from build123d import *

# Parameters (mm, degrees)
EXTRUDE_1_DEPTH      = 10.8
SKETCH_2_R           = 1
EXTRUDE_2_DEPTH      = 0.8
SKETCH_3_W           = 1.7
SKETCH_3_H           = 8.1
CUT_EXTRUDE_1_DEPTH  = 17.8
EXTRUDE_START        = -4.5
EXTRUDE_3_DEPTH      = 4.5
SKETCH_5_W           = 8.4
SKETCH_5_H           = 0.05
CUT_EXTRUDE_2_DEPTH  = 1
SKETCH_6_R           = 1
CUT_EXTRUDE_3_DEPTH  = 8
CUT_EXTRUDE_4_DEPTH  = 1.2
SKETCH_8_W           = 2.8
SKETCH_8_H           = 0.608363533
EXTRUDE_4_DEPTH      = 0.1
EXTRUDE_START_2      = 2.5
EXTRUDE_5_DEPTH      = 2.5
SKETCH_10_W          = 8.4
SKETCH_10_H          = 1.7
CUT_EXTRUDE_5_DEPTH  = 0.05
FILLET_1_R           = 1.4
SKETCH_11_W          = 0.05
SKETCH_11_H          = 5.83834946
SKETCH_11_H_2        = 5.828769054
CUT_EXTRUDE_8_DEPTH  = 0.05
CUT_EXTRUDE_9_DEPTH  = 4
SKETCH_13_W          = 0.5
SKETCH_13_H          = 5.54
EXTRUDE_6_DEPTH      = 1.45
FILLET_2_R           = 1
CUT_EXTRUDE_START    = -8.12
CUT_EXTRUDE_10_DEPTH = 8.12
SKETCH_15_W          = 3
SKETCH_15_H          = 0.25
CUT_EXTRUDE_11_DEPTH = 8.12
SKETCH_16_W          = 0.5
SKETCH_16_H          = 0.25
EXTRUDE_7_DEPTH      = 3
FILLET_3_R           = 0.5
FILLET_4_R           = 0.75


with BuildPart() as part:
    # Эскиз1 → Бобышка-Вытянуть1 (new body)
    with BuildSketch(Plane.XY):
        Polygon((7.4, 0), (8.4, 1), (8.4, 12.6), (0, 12.6), (0, 1), (1, 0), align=None)
    extrude(amount=EXTRUDE_1_DEPTH)

    # Эскиз2 → Бобышка-Вытянуть2 (add)
    with BuildSketch(Plane(origin=(0, 0, 0), x_dir=(-1, 0, 0), z_dir=(0, 0, -1))):
        with Locations((-4.2, 10.3)):
            Circle(SKETCH_2_R)
        with Locations((-4.2, 3.9)):
            Circle(SKETCH_2_R)
    extrude(amount=EXTRUDE_2_DEPTH)

    # Эскиз3 → Вырез-Вытянуть1 (cut)
    with BuildSketch(Plane(origin=(8.4, 0, 0), x_dir=(0, 0, -1), z_dir=(1, 0, 0))):
        with Locations((-4.75, 4.05)):
            Rectangle(SKETCH_3_W, SKETCH_3_H)
    extrude(amount=-CUT_EXTRUDE_1_DEPTH, mode=Mode.SUBTRACT)

    # Эскиз4 → Бобышка-Вытянуть3 (add)
    with BuildSketch(Plane(origin=(0, 12.6, 0), x_dir=(1, 0, 0), z_dir=(0, 1, 0)).offset(EXTRUDE_START)):
        with BuildLine():
            Line((9.1, -10.8), (-0.7, -10.8))
            Line((-0.7, -10.8), (-0.7, -2.8))
            ThreePointArc((-0.7, -2.8), (-0.992893219, -2.092893219), (-1.7, -1.8))
            Line((-1.7, -1.8), (-5.9, -1.8))
            Line((-5.9, -1.8), (-5.9, 0))
            Line((-5.9, 0), (14.3, 0))
            Line((14.3, 0), (14.3, -1.8))
            Line((14.3, -1.8), (10.1, -1.8))
            ThreePointArc((10.1, -1.8), (9.392893219, -2.092893219), (9.1, -2.8))
            Line((9.1, -2.8), (9.1, -10.8))
        make_face()
    extrude(amount=EXTRUDE_3_DEPTH)

    # Эскиз5 → Вырез-Вытянуть2 (cut)
    with BuildSketch(Plane.XY.offset(10.8)):
        with Locations((4.2, 8.075)):
            Rectangle(SKETCH_5_W, SKETCH_5_H)
    extrude(amount=-CUT_EXTRUDE_2_DEPTH, mode=Mode.SUBTRACT)

    # Эскиз6 → Вырез-Вытянуть3 (cut)
    with BuildSketch(Plane.XY.offset(10.8)):
        with Locations((4.2, 4)):
            Circle(SKETCH_6_R)
    extrude(amount=-CUT_EXTRUDE_3_DEPTH, mode=Mode.SUBTRACT)

    # Эскиз7 → Вырез-Вытянуть4 (cut)
    with BuildSketch(Plane(origin=(0, 12.6, 0), x_dir=(1, 0, 0), z_dir=(0, 1, 0))):
        with BuildLine():
            Line((8.6, 0), (8.6, -7.112411136))
            ThreePointArc((8.6, -7.112411136), (8.468198052, -7.430609188), (8.15, -7.562411136))
            Line((8.15, -7.562411136), (7.983405928, -7.562411136))
            ThreePointArc((7.983405928, -7.562411136), (7.691564003, -7.454943311), (7.539115931, -7.183870205))
            Line((7.539115931, -7.183870205), (7.049736844, -4.141202068))
            ThreePointArc((7.049736844, -4.141202068), (6.710963351, -3.53881739), (6.062425739, -3.3))
            Line((6.062425739, -3.3), (2.361664993, -3.3))
            ThreePointArc((2.361664993, -3.3), (1.71573807, -3.536600753), (1.37546474, -4.13444318))
            Line((1.37546474, -4.13444318), (0.863036378, -7.186911705))
            ThreePointArc((0.863036378, -7.186911705), (0.709913379, -7.455940797), (0.419246264, -7.562411136))
            Line((0.419246264, -7.562411136), (0.25, -7.562411136))
            ThreePointArc((0.25, -7.562411136), (-0.068198052, -7.430609188), (-0.2, -7.112411136))
            Line((-0.2, -7.112411136), (-0.2, 0))
            Line((-0.2, 0), (8.6, 0))
        make_face()
        with BuildLine():
            Line((4.2, -10.8), (5.6, -10.8))
            Line((5.6, -10.8), (5.6, -5.056380156))
            ThreePointArc((5.6, -5.056380156), (5.453553391, -4.702826765), (5.1, -4.556380156))
            Line((5.1, -4.556380156), (3.3, -4.556380156))
            ThreePointArc((3.3, -4.556380156), (2.946446609, -4.702826765), (2.8, -5.056380156))
            Line((2.8, -5.056380156), (2.8, -10.8))
            Line((2.8, -10.8), (4.2, -10.8))
        make_face()
    extrude(amount=-CUT_EXTRUDE_4_DEPTH, mode=Mode.SUBTRACT)

    # Эскиз8 → Бобышка-Вытянуть4 (add)
    with BuildSketch(Plane(origin=(0, 11.4, 0), x_dir=(1, 0, 0), z_dir=(0, 1, 0))):
        with Locations((4.2, -10.495818233)):
            Rectangle(SKETCH_8_W, SKETCH_8_H)
    extrude(amount=EXTRUDE_4_DEPTH)

    # Эскиз9 → Бобышка-Вытянуть5 (add)
    with BuildSketch(Plane.XZ.offset(-8.1).offset(EXTRUDE_START_2)):
        with BuildLine():
            Line((0, 0), (0, 3.7))
            Line((0, 3.7), (-0.7, 3.7))
            Line((-0.7, 3.7), (-0.7, 2.8))
            ThreePointArc((-0.7, 2.8), (-0.992893219, 2.092893219), (-1.7, 1.8))
            Line((-1.7, 1.8), (-5.9, 1.8))
            Line((-5.9, 1.8), (-5.9, 0))
            Line((-5.9, 0), (0, 0))
        make_face()
        with BuildLine():
            Line((14.3, 0), (8.4, 0))
            Line((8.4, 0), (8.4, 3.7))
            Line((8.4, 3.7), (9.1, 3.7))
            Line((9.1, 3.7), (9.1, 2.8))
            ThreePointArc((9.1, 2.8), (9.392893219, 2.092893219), (10.1, 1.8))
            Line((10.1, 1.8), (14.3, 1.8))
            Line((14.3, 1.8), (14.3, 0))
        make_face()
    extrude(amount=-EXTRUDE_5_DEPTH)

    # Эскиз10 → Вырез-Вытянуть5 (cut)
    with BuildSketch(Plane.XZ.offset(-8.1)):
        with Locations((4.2, 4.75)):
            Rectangle(SKETCH_10_W, SKETCH_10_H)
    extrude(amount=-CUT_EXTRUDE_5_DEPTH, mode=Mode.SUBTRACT)

    # Скругление1
    fillet_1_edges = [part.edges().sort_by_distance(p)[0] for p in [
        (-5.9, 5.6, 0.9),
        (14.3, 5.6, 0.9),
        (14.3, 12.6, 0.9),
        (-5.9, 12.6, 0.9),
    ]]
    fillet(fillet_1_edges, radius=FILLET_1_R)

    # Эскиз11 → Вырез-Вытянуть8 (cut)
    with BuildSketch(Plane(origin=(0, 0, 0), x_dir=(-1, 0, 0), z_dir=(0, 0, -1))):
        with Locations((-8.375, 8.48082527)):
            Rectangle(SKETCH_11_W, SKETCH_11_H)
        with Locations((-0.025, 8.485615473)):
            Rectangle(SKETCH_11_W, SKETCH_11_H_2)
    extrude(amount=-CUT_EXTRUDE_8_DEPTH, mode=Mode.SUBTRACT)

    # Эскиз12 → Вырез-Вытянуть9 (cut)
    with BuildSketch(Plane(origin=(0, 0, 0), x_dir=(-1, 0, 0), z_dir=(0, 0, -1))):
        with BuildLine():
            Line((1.9, 9), (1.9, 10.4))
            ThreePointArc((1.9, 10.4), (3.3, 11.8), (4.7, 10.4))
            Line((4.7, 10.4), (4.7, 9))
            ThreePointArc((4.7, 9), (4.690102856, 8.833825246), (4.660551359, 8.67))
            ThreePointArc((4.660551359, 8.67), (3.3, 6.94), (1.939448641, 8.67))
            ThreePointArc((1.939448641, 8.67), (1.909897144, 8.833825246), (1.9, 9))
        make_face()
        with BuildLine():
            Line((-10.3, 10.4), (-10.3, 9))
            ThreePointArc((-10.3, 9), (-10.309897144, 8.833825246), (-10.339448641, 8.67))
            ThreePointArc((-10.339448641, 8.67), (-11.7, 6.94), (-13.060551359, 8.67))
            ThreePointArc((-13.060551359, 8.67), (-13.090102856, 8.833825246), (-13.1, 9))
            Line((-13.1, 9), (-13.1, 10.4))
            ThreePointArc((-13.1, 10.4), (-11.7, 11.8), (-10.3, 10.4))
        make_face()
    extrude(amount=-CUT_EXTRUDE_9_DEPTH, mode=Mode.SUBTRACT)

    # Эскиз13 → Бобышка-Вытянуть6 (add)
    with BuildSketch(Plane(origin=(0, 11.4, 0), x_dir=(1, 0, 0), z_dir=(0, 1, 0))):
        with Locations((5.47, 0.23)):
            Rectangle(SKETCH_13_W, SKETCH_13_H)
        with Locations((8.01, 0.23)):
            Rectangle(SKETCH_13_W, SKETCH_13_H)
        with Locations((2.93, 0.23)):
            Rectangle(SKETCH_13_W, SKETCH_13_H)
        with Locations((0.39, 0.23)):
            Rectangle(SKETCH_13_W, SKETCH_13_H)
    extrude(amount=EXTRUDE_6_DEPTH)

    # Скругление2
    fillet_2_edges = [part.edges().sort_by_distance(p)[0] for p in [
        (5.47, 12.85, 2.54),
        (2.93, 12.85, 2.54),
        (0.39, 12.85, 2.54),
        (8.01, 12.85, 2.54),
    ]]
    fillet(fillet_2_edges, radius=FILLET_2_R)

    # Эскиз14 → Вырез-Вытянуть10 (cut)
    with BuildSketch(Plane.ZY.offset(-0.14).offset(CUT_EXTRUDE_START)):
        with BuildLine():
            Line((-3, 12.6), (1.54, 12.6))
            ThreePointArc((1.54, 12.6), (2.070330086, 12.380330086), (2.29, 11.85))
            Line((2.29, 11.85), (2.29, 11.4))
            Line((2.29, 11.4), (-3, 11.4))
            Line((-3, 11.4), (-3, 12.6))
        make_face()
    extrude(amount=CUT_EXTRUDE_10_DEPTH, mode=Mode.SUBTRACT)

    # Эскиз15 → Вырез-Вытянуть11 (cut)
    with BuildSketch(Plane(origin=(8.26, 0, 0), x_dir=(0, 0, -1), z_dir=(1, 0, 0)).offset(CUT_EXTRUDE_START)):
        with Locations((1.5, 12.725)):
            Rectangle(SKETCH_15_W, SKETCH_15_H)
    extrude(amount=CUT_EXTRUDE_11_DEPTH, mode=Mode.SUBTRACT)

    # Эскиз16 → Бобышка-Вытянуть7 (add)
    with BuildSketch(Plane(origin=(0, 12.85, 0), x_dir=(1, 0, 0), z_dir=(0, 1, 0))):
        with Locations((8.01, -0.125)):
            Rectangle(SKETCH_16_W, SKETCH_16_H)
        with Locations((5.47, -0.125)):
            Rectangle(SKETCH_16_W, SKETCH_16_H)
        with Locations((2.93, -0.125)):
            Rectangle(SKETCH_16_W, SKETCH_16_H)
        with Locations((0.39, -0.125)):
            Rectangle(SKETCH_16_W, SKETCH_16_H)
    extrude(amount=EXTRUDE_7_DEPTH)

    # Скругление3
    fillet_3_edges = [part.edges().sort_by_distance(p)[0] for p in [
        (8.01, 12.85, 0.25),
        (5.47, 12.85, 0.25),
        (2.93, 12.85, 0.25),
        (0.39, 12.85, 0.25),
    ]]
    fillet(fillet_3_edges, radius=FILLET_3_R)

    # Скругление4
    fillet_4_edges = [part.edges().sort_by_distance(p)[0] for p in [
        (5.47, 12.6, 0),
        (2.93, 12.6, 0),
        (0.39, 12.6, 0),
        (8.01, 12.6, 0),
    ]]
    fillet(fillet_4_edges, radius=FILLET_4_R)


solid = part.part
Part model, mm, in its own coordinate system. A direction names the side the tool comes from. Round coordinates to 2 decimals unless told otherwise and drop trailing zeros. Write each loop counter-clockwise with the first axis right and the second up, starting at its lowest first coordinate (ties: lowest second). Pieces come first, ordered by that corner, then holes. Notation, with made-up numbers: (8.25, 17.25) - (65.25, 17.25) arc R23 cw to (65.25, 47.25) - close; hole circle Ø3 at (-25.5, 49.25). An arc over 180 degrees is marked (long way). Use CSV: the item, a comma, the result in double quotes.
Item 1: Flat gauge pins, fed straight in: P1, Ø6, axis at x = 6, z = 5, coming from the +Y side; P2, Ø0.5, axis at x = 3, z = 5, coming from the -Y side; P3, Ø4, axis at x = 0.5, z = 4.5, coming from the +Y side; P4, Ø2.5, axis at x = -3.3, y = 8.34, coming from the -Z side. Where does each tip first touch, or does it go through?
Results list:
P1,"stops at y = 12.73"
P2,"stops at y = 8.15"
P3,"stops at y = 12.6"
P4,"passes through"
Item 2: Slice it at B-B, the plane y = 10.75. Count the separate pieces of the cut face and the enclosed holes in it, then the cut area to 3 significant figures.
Results list:
separate pieces,"3"
enclosed holes,"0"
area,"117 mm²"
Item 3: Tool access for faces 4 (the flat face through (14, 9, 1.8)), 5 (the flat face through (4, 11.4, 7)), 6 (the flat face through (-1.7, 9.1, 0)), 7 (the flat face through (-4.7, 10, 1)), 8 (the cylindrical face through (5, 3.3, -0.4)): list every direction of +Z, -Z, +X, -X, +Y, -Y with a clear straight run to the whole face (end or side of a thin tool).
Results list:
face 4,"+Z, +X, +Y, -Y"
face 5,"+Y"
face 6,"-Z, -X, +Y, -Y"
face 7,"+Z, -Z"
face 8,"-Z"
Item 4: Wall check: L1, parallel to X at y = 8.34, z = 1.2; L2, parallel to Y at x = 4.2, z = 3.55; L3, parallel to Z at x = 1.5, y = 1. Give the ranges that are in metal, low to high.
Results list:
L1,"x = -5.9 to -4.7, -1.9 to 10.3, 13.1 to 14.3"
L2,"y = 0 to 3, 5 to 12.6"
L3,"z = 0 to 3.9, 5.6 to 10.8"
Item 5: Slice it at C-C, the plane x = -3.3. Write the cut outline in (y, z), then the cut area to 3 significant figures.
Results list:
outline,"(5.6, 0) - (6.94, 0) - (6.94, 1.8) - (5.6, 1.8) - close; (11.8, 0) - (12.6, 0) - (12.6, 1.8) - (11.8, 1.8) - close"
area,"3.85 mm²"
Item 6: Slice it at D-D, the plane y = 4.5. Write the cut outline in (x, z).
Results list:
outline,"(0, 0) - (3.4, 0) - (3.4, -0.8) - (5, -0.8) - (5, 0) - (8.4, 0) - (8.4, 3.9) - (5.07, 3.9) - (5.07, 2.8) - (3.33, 2.8) - (3.33, 3.9) - (0, 3.9) - close; (0, 5.6) - (3.33, 5.6) - (3.33, 10.8) - (0, 10.8) - close; (5.07, 5.6) - (8.4, 5.6) - (8.4, 10.8) - (5.07, 10.8) - close"
Item 7: Pull direction Y, two halves, no side cores. Call faces 1 (the flat face through (8.4, 4, 2)), 2 (the flat face through (4, 0, 2)), 3 (the flat face through (4, 11.4, 3)): pulls with the +Y half, pulls with the -Y half, needs draft (parallel to the pull), parting line crosses it, or undercut.
Results list:
face 1,"needs draft"
face 2,"pulls with the -Y half"
face 3,"undercut"
